from build123d import *

# Parameters (mm, degrees)
SKETCH1_W           = 20
SKETCH1_H           = 96
BOSS_EXTRUDE1_DEPTH = 2
SKETCH2_R           = 4
SKETCH2_R_2         = 1.75
SKETCH2_R_3         = 3.75
CUT_EXTRUDE1_DEPTH  = 99.081598682
CHAMFER1_SIZE       = 2


with BuildPart() as part:
    # Sketch1 → Boss-Extrude1 (new body)
    with BuildSketch(Plane(origin=(0, 0, 0), x_dir=(0, 0, -1), z_dir=(1, 0, 0))):
        with Locations((10, 48)):
            Rectangle(SKETCH1_W, SKETCH1_H)
    extrude(amount=BOSS_EXTRUDE1_DEPTH)

    # Sketch2 → Cut-Extrude1 (cut, through all)
    with BuildSketch(Plane(origin=(2, 0, 0), x_dir=(0, 0, -1), z_dir=(1, 0, 0))):
        with Locations((10, 85.5)):
            Circle(SKETCH2_R)
        with Locations((10, 52.75)):
            Circle(SKETCH2_R_2)
        with Locations((10, 20)):
            Circle(SKETCH2_R_3)
    extrude(amount=-CUT_EXTRUDE1_DEPTH, mode=Mode.SUBTRACT)

    # Chamfer1
    chamfer1_edges = [part.edges().sort_by_distance(p)[0] for p in [
        (1, 96, 0),
        (1, 96, -20),
        (1, 0, -20),
        (1, 0, 0),
    ]]
    chamfer(chamfer1_edges, length=CHAMFER1_SIZE)


solid = part.part
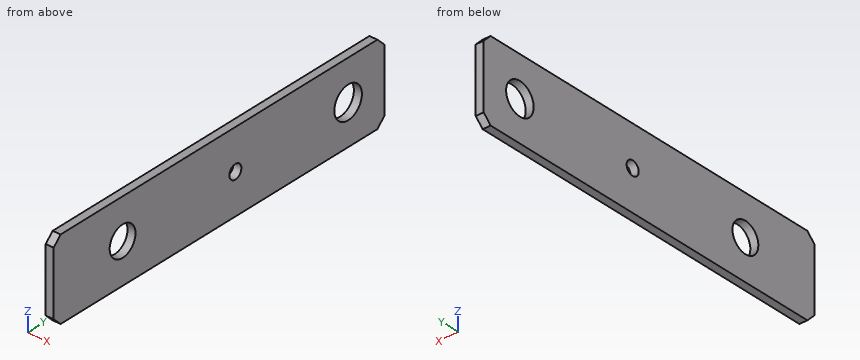
Model file for the job. Use its own axes, mm. Give positions to 0.01 mm unless a question says otherwise; leave off trailing zeros. Loops run counter-clockwise (first coordinate to the right, second up) from the corner with the lowest first, then second, coordinate; pieces in that order, holes last. Notation, with made-up numbers: (-3.5, 68) -> (34.5, 68) arc R21 ccw to (34.5, 73) -> close; hole circle Ø3 at (-29.75, 3). An arc over 180 degrees is marked (long way). Use a Markdown table: item, result. Add a question column.
(1) Drop a flat-ended pin along its axis: pin 1 Ø1 at (y, z) = (68, -10.5) entering from -X. Give the stop position or say it passes through.
(2) Slice it at A-A on y = 20. List the corners of the cut face in (x, z), and give its area (3 significant figures).
(3) Slice it at C-C on x = 1.3. List the corners of the cut face in (y, z).
(4) Slice it at D-D on y = 52.75. List the corners of the cut face in (x, z), and give its area (3 significant figures).
(5) Wall check: line 1 along Y through (x, z) = (0.9, -10); line 2 along Y through (x, z) = (1.45, -12.25); line 3 along Z through (x, y) = (0.2, 53.5). Give the ranges that are in metal, low to high.
(6) Slice it at B-B on z = -10. List the corners of the cut face in (x, y).
Filled sheet:
| question | item | result |
|---|---|---|
| 1 | pin 1 | x = 0 |
| 2 | outline | (0, -20) -> (2, -20) -> (2, -13.75) -> (0, -13.75) -> close; (0, -6.25) -> (2, -6.25) -> (2, 0) -> (0, 0) -> close |
| 2 | area | 25.0 mm2 |
| 3 | outline | (0, -18) -> (2, -20) -> (94, -20) -> (96, -18) -> (96, -2) -> (94, 0) -> (2, 0) -> (0, -2) -> close; hole circle Ø7.5 at (20, -10); hole circle Ø3.5 at (52.75, -10); hole circle Ø8 at (85.5, -10) |
| 4 | outline | (0, -20) -> (2, -20) -> (2, -11.75) -> (0, -11.75) -> close; (0, -8.25) -> (2, -8.25) -> (2, 0) -> (0, 0) -> close |
| 4 | area | 33.0 mm2 |
| 5 | line 1 | 0 to 16.25, 23.75 to 51, 54.5 to 81.5, 89.5 to 96 |
| 5 | line 2 | 0 to 17, 23 to 82.19, 88.81 to 96 |
| 5 | line 3 | -20 to -11.58, -8.42 to 0 |
| 6 | outline | (0, 0) -> (2, 0) -> (2, 16.25) -> (0, 16.25) -> close; (0, 23.75) -> (2, 23.75) -> (2, 51) -> (0, 51) -> close; (0, 54.5) -> (2, 54.5) -> (2, 81.5) -> (0, 81.5) -> close; (0, 89.5) -> (2, 89.5) -> (2, 96) -> (0, 96) -> close |
